from build123d import *

# Parameters (mm, degrees)
SKETCH2_W           = 14
SKETCH2_H           = 5.5
BOSS_EXTRUDE1_DEPTH = 8
BOSS_EXTRUDE2_START = 4
BOSS_EXTRUDE2_DEPTH = 3


with BuildPart() as part:
    # Sketch1 → Revolve1 (revolve)
    with BuildSketch(Plane.XY, mode=Mode.PRIVATE) as revolve1_sk:
        with BuildLine():
            Line((9.5, 0), (11, 0))
            Line((11, 0), (11, 0.6))
            Line((11, 0.6), (8.75, 2))
            Line((8.75, 2), (7.5, 2))
            Line((7.5, 2), (7.5, 3.6))
            Line((7.5, 3.6), (6.5, 3.6))
            ThreePointArc((6.5, 3.6), (3.259601203, 3.225184366), (0, 3.1))
            Line((0, 3.1), (0, -17.4))
            Line((0, -17.4), (9.5, -17.4))
            Line((9.5, -17.4), (9.5, 0))
        make_face()
    revolve(revolve1_sk.sketch.rotate(Axis((0, 3.6, 0), (0, 1, 0)), 90), axis=Axis((0, 3.6, 0), (0, 1, 0)))

    # Sketch2 → Boss-Extrude1 (add)
    with BuildSketch(Plane.XZ.offset(17.4)):
        Rectangle(SKETCH2_W, SKETCH2_H)
    extrude(amount=BOSS_EXTRUDE1_DEPTH)

    # Sketch3 → Boss-Extrude2 (add)
    with BuildSketch(Plane.XZ.offset(BOSS_EXTRUDE2_START)):
        Polygon((0, 12.701705922), (-11, 6.350852961), (-11, -6.350852961), (0, -12.701705922), (11, -6.350852961), (11, 6.350852961), align=None)
    extrude(amount=BOSS_EXTRUDE2_DEPTH)


solid = part.part
Geometry: final body of the model. Coordinates: model frame, mm. A direction names the side the tool comes from. Give positions to 0.01 mm unless a question says otherwise; leave off trailing zeros. Write each loop counter-clockwise with the first axis right and the second up, starting at its lowest first coordinate (ties: lowest second). Pieces come first, ordered by that corner, then holes.
(1) Mould query, pull axis Y, two halves, no side actions, for faces 4 (the cylindrical face through (9.274, -1.972, 2.059)), 5 (the cylindrical face through (10.74, 0.3, 2.38)), 6 (the flat face through (-3, 3.6, 6)). Classes: released by +Y, released by -Y, zero draft, split by the parting line, or undercut.
(2) Access query for faces 1 (the flat face through (0, 0, -10)), 2 (the flat face through (-7, 2, 4)), 3 (the flat face through (0, -21, 2.75)). Directions: +Z, -Z, +X, -X, +Y, -Y. A direction counts if a zero-diameter tool reaches every point of the face in a straight line with its end or side. Return the directions, or none.
(3) Cut plane D-D, the plane y = -23. Return loops of the section in (x, z).
(4) First-contact query: P1, Ø5, axis at x = 8, z = -0.5, coming from the +Y side; P2, Ø1.6, axis at y = -20, z = 0.5, coming from the +X side; P3, Ø1, axis at x = -5, y = -10.5, coming from the -Z side; P4, Ø4.5, axis at y = -23, z = 1, coming from the -X side. Flat tips, straight axial feed; report the tip coordinate or a pass-through.
(5) Cut plane B-B, the plane y = -5.75. Return loops of the section in (x, z).
(6) Cut plane C-C, the plane y = -12.25. Return loops of the section in (x, z).
(7) Ray query, line 1 (Y direction, x = -4.25, z = -5.25); line 2 (X direction, y = -24, z = -2); line 3 (X direction, y = -13, z = 0). Return the intervals inside material, ascending.
(8) Cut plane A-A, the plane z = 0. Return loops of the section in (x, y), then the cut area to 3 significant figures.
Values follow:
1. face 4: undercut
1. face 5: zero draft
1. face 6: released by +Y
2. face 1: none
2. face 2: +Y
2. face 3: +Z, +X, -X, -Y
3. outline: (-7, -2.75) - (7, -2.75) - (7, 2.75) - (-7, 2.75) - close
4. P1: stops at y = 3.6
4. P2: stops at x = 7
4. P3: stops at z = -8.37
4. P4: stops at x = -7
5. outline: (-11, -6.35) - (0, -12.7) - (11, -6.35) - (11, 6.35) - (0, 12.7) - (-11, 6.35) - close
6. outline: circle Ø19 at (0, 0)
7. line 1: y = -17.4 to 3.6
7. line 2: x = -7 to 7
7. line 3: x = -9.5 to 9.5
8. outline: (-11, -7) - (-9.5, -7) - (-9.5, -17.4) - (-7, -17.4) - (-7, -25.4) - (7, -25.4) - (7, -17.4) - (9.5, -17.4) - (9.5, -7) - (11, -7) - (11, -4) - (9.5, -4) - (9.5, 0) - (11, 0) - (11, 0.6) - (8.75, 2) - (7.5, 2) - (7.5, 3.6) - (6.5, 3.6) arc R42.5 cw to (-6.5, 3.6) - (-7.5, 3.6) - (-7.5, 2) - (-8.75, 2) - (-11, 0.6) - (-11, 0) - (-9.5, 0) - (-9.5, -4) - (-11, -4) - close
8. area: 512 mm2
